Check sheet for the modelled part. Datum: model origin and axes. Units: mm. A direction names the side the tool comes from. Coordinates: 2 decimals unless noted, no trailing zeros. Order: outer loops, then holes, each group sorted by start corner. A loop starts at its lowest first (then second) coordinate and runs counter-clockwise, first axis right, second up.
from build123d import *

# Parameters (mm, degrees)
BASE_EXTRUDE_DEPTH = 12.7
CIRPATTERN1_COUNT  = 2
LPATTERN1_COUNT    = 2
LPATTERN1_PITCH    = 82.55


with BuildPart() as part:
    # Sketch1 → Base-Extrude (new, symmetric)
    with BuildSketch(Plane.XY):
        with BuildLine():
            Line((-41.275, 15.875), (-41.275, -17.9451))
            ThreePointArc((-41.275, -17.9451), (-40.486414298, -19.848914298), (-38.5826, -20.6375))
            Line((-38.5826, -20.6375), (-2.6924, -20.6375))
            ThreePointArc((-2.6924, -20.6375), (-0.788585702, -19.848914298), (0, -17.9451))
            Line((0, -17.9451), (0, 15.875))
            ThreePointArc((0, 15.875), (-4.7625, 20.6375), (-9.525, 15.875))
            Line((-9.525, 15.875), (-9.525, 14.83995))
            ThreePointArc((-9.525, 14.83995), (-8.1788, 13.49375), (-6.8326, 14.83995))
            Line((-6.8326, 14.83995), (-6.8326, 15.875))
            ThreePointArc((-6.8326, 15.875), (-4.7625, 17.9451), (-2.6924, 15.875))
            Line((-2.6924, 15.875), (-2.6924, -17.9451))
            Line((-2.6924, -17.9451), (-38.5826, -17.9451))
            Line((-38.5826, -17.9451), (-38.5826, 15.875))
            ThreePointArc((-38.5826, 15.875), (-36.5125, 17.9451), (-34.4424, 15.875))
            Line((-34.4424, 15.875), (-34.4424, 14.83995))
            ThreePointArc((-34.4424, 14.83995), (-33.0962, 13.49375), (-31.75, 14.83995))
            Line((-31.75, 14.83995), (-31.75, 15.875))
            ThreePointArc((-31.75, 15.875), (-36.5125, 20.6375), (-41.275, 15.875))
        make_face()
    base_extrude = extrude(amount=BASE_EXTRUDE_DEPTH, both=True)

    # CirPattern1: Base-Extrude ×2 about axis
    cirpattern1_axis = Axis((0, 0, 0), (0, 0, 1))
    for i in range(1, CIRPATTERN1_COUNT):
        add(base_extrude.rotate(cirpattern1_axis, i * 360 / CIRPATTERN1_COUNT))

    # LPattern1: Base-Extrude ×2
    with Locations(*[(i * LPATTERN1_PITCH, 0, 0) for i in range(1, LPATTERN1_COUNT)]):
        add(base_extrude)


solid = part.part
(1) Thickness scan on probe 1 along X at (y, z) = (0, 9.5) (3 decimals); probe 2 along X at (y, z) = (18.5, 2); probe 3 along Y at (x, z) = (-24.5, 4.5). Record the ranges inside material, lowest first.
Filled in:
probe 1: x = -41.275 to -38.583, -2.692 to 2.692, 38.583 to 43.967, 79.858 to 82.55
probe 2: x = -40.49 to -32.54, -8.74 to -0.79, 0.06 to 41.22, 42.06 to 50.01, 73.81 to 81.76
probe 3: y = -20.64 to -17.95
(2) Go/stop test with flat-tipped pins: P1, Ø1.7, axis at y = 17, z = -1.5, coming from the +X side; P2, Ø1.7, axis at y = 17, z = -1.5, coming from the -X side; P3, Ø12, axis at x = 54, y = 5.5, coming from the +Z side; P4, Ø8, axis at x = 30.5, z = -6.5, coming from the -Y side. Record where each tip stops, or that it passes through.
Filled in:
P1: stops at x = 82.54
P2: stops at x = -41.27
P3: passes through
P4: stops at y = -20.19
(3) Cross-section at C-C (x = 30.5). Enter the section's corners in (y, z).
Filled in:
outline: (17.95, -12.7) - (20.64, -12.7) - (20.64, 12.7) - (17.95, 12.7) - close
(4) Cross-section at B-B (x = -8). Enter the section's corners in (y, z), and give its area (3 significant figures).
Filled in:
outline: (-20.64, -12.7) - (-17.95, -12.7) - (-17.95, 12.7) - (-20.64, 12.7) - close; (13.51, -12.7) - (19.37, -12.7) - (19.37, 12.7) - (13.51, 12.7) - close
area: 217 mm2
(5) Release check for a two-part mould opening along Y. For faces 5 (the cylindrical face through (77.892, 20.636, 0.178)), 6 (the cylindrical face through (74.342, 13.494, 0.178)), 7 (the flat face through (62, -20.638, 0)) record: +Y half, -Y half, draft (parallel to the pull), parting line (faces both ways), or undercut.
Filled in:
face 5: +Y half
face 6: undercut
face 7: -Y half
(6) Tool access check on faces 1 (the cylindrical face through (0.81, 19.87, 0.18)), 2 (the flat face through (41.275, 17.1, 0.2)), 3 (the flat face through (43.967, -1, 0)), 4 (the cylindrical face through (-40.507, -19.828, 0.178)). Record the directions out of +Z, -Z, +X, -X, +Y, -Y that give a thin tool (end or side, any length) a straight path to the whole face; none if there is none.
Filled in:
face 1: +Z, -Z, +Y
face 2: none
face 3: +Z, -Z
face 4: +Z, -Z, -X, -Y
(7) Cross-section at A-A (y = 2). Enter the section's corners in (x, z) (3 decimals).
Filled in:
outline: (-41.275, -12.7) - (-38.583, -12.7) - (-38.583, 12.7) - (-41.275, 12.7) - close; (-2.692, -12.7) - (2.692, -12.7) - (2.692, 12.7) - (-2.692, 12.7) - close; (38.583, -12.7) - (43.967, -12.7) - (43.967, 12.7) - (38.583, 12.7) - close; (79.858, -12.7) - (82.55, -12.7) - (82.55, 12.7) - (79.858, 12.7) - close
